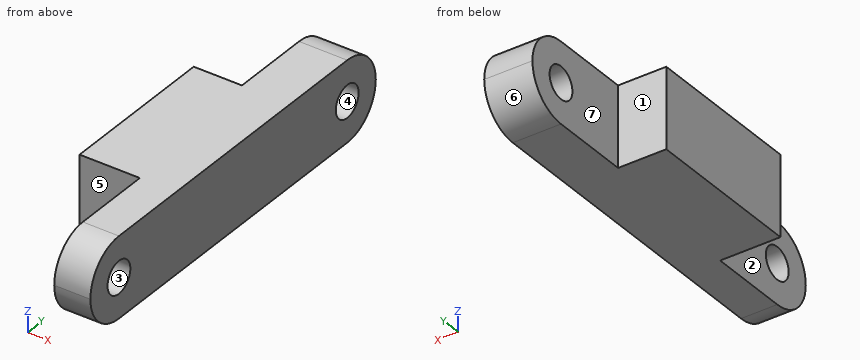
from build123d import *

# Parameters (mm, degrees)
SKETCH1_W           = 12
SKETCH1_H           = 50
BOSS_EXTRUDE1_DEPTH = 10
SKETCH2_W           = 7.5
SKETCH2_H           = 15
SKETCH2_W_2         = 6
CUT_EXTRUDE1_DEPTH  = 10
SKETCH3_R           = 2
CUT_EXTRUDE2_DEPTH  = 10
FILLET1_R           = 5


with BuildPart() as part:
    # Sketch1 → Boss-Extrude1 (new body)
    with BuildSketch(Plane.XY):
        Rectangle(SKETCH1_W, SKETCH1_H)
    extrude(amount=BOSS_EXTRUDE1_DEPTH)

    # Sketch2 → Cut-Extrude1 (cut)
    with BuildSketch(Plane.XY.offset(10)):
        with Locations((-2.25, -17.5)):
            Rectangle(SKETCH2_W, SKETCH2_H)
        with Locations((-3, 17.5)):
            Rectangle(SKETCH2_W_2, SKETCH2_H)
    extrude(amount=-CUT_EXTRUDE1_DEPTH, mode=Mode.SUBTRACT)

    # Sketch3 → Cut-Extrude2 (cut)
    with BuildSketch(Plane.ZY):
        with Locations(Location((5, 20, 0), (0, 0, 270))):
            Circle(SKETCH3_R)
        with Locations(Location((5, -20, 0), (0, 0, 270))):
            Circle(SKETCH3_R)
    extrude(amount=-CUT_EXTRUDE2_DEPTH, mode=Mode.SUBTRACT)

    # Fillet1
    fillet1_edges = [part.edges().sort_by_distance(p)[0] for p in [
        (3.75, -25, 0),
        (3.75, -25, 10),
        (3, 25, 0),
        (3, 25, 10),
    ]]
    fillet(fillet1_edges, radius=FILLET1_R - 0.0001)  # a hair under: the kernel refuses the full size


solid = part.part
Work out the finished part from the listing and answer in its coordinate system (mm). Face numbers are marked on the shaded views. A direction names the side the tool comes from. Coordinates: 2 decimals unless noted, no trailing zeros. Loops run counter-clockwise (first coordinate to the right, second up) from the corner with the lowest first, then second, coordinate; pieces in that order, holes last. Notation, with made-up numbers: M 48,23.5 L 65,23.5 A21 cw 65,27.5 Z; hole C 66,-26 d4. An arc over 180 degrees is marked long. Answer in a Markdown table with one row per item. Add a question column.
1. A tool of negligible diameter and unlimited length cuts with its end or side. For the marked faces 5, 6 and 7, from which of +Z, -Z, +X, -X, +Y, -Y can it reach the whole face along a straight path? Write none if from no direction.
2. Find section A-A, the plane x = 3. State how many separate pieces and enclosed holes the cut face has, then the cut area to 3 significant figures.
3. Find section C-C, the plane y = -19. Write down the section's boundary in (x, z).
4. Consider L1, parallel to Z at x = 1.75, y = 20; L2, parallel to Y at x = 2, z = 4; L3, parallel to Y at x = -2.5, z = 5.75. Determine where each line is inside the solid, lowest interval first.
5. Flat-ended cylindrical pins translate along their axes: P1, Ø4, axis at x = -2, z = 3, coming from the -Y side; P2, Ø3.5, axis at y = -20, z = 5, coming from the +X side; P3, Ø3, axis at x = -4, z = 7, coming from the +Y side. Find the tip coordinate at first contact, or state that the pin passes through.
6. Find section D-D, the plane x = -5.5. Write down the section's boundary in (y, z).
7. The mould has two halves that part along Y. Classify the marked faces 1, 2, 3 and 4: pulls with the +Y half, pulls with the -Y half, needs draft (parallel to the pull), parting line crosses it, or undercut.
8. Find section B-B, the plane z = 3.75. Write down the section's boundary in (x, y), then the cut area to 3 significant figures.
Reported:
| question | item | result |
|---|---|---|
| 1 | face 5 | +Z, -Z, -X, -Y |
| 1 | face 6 | -Z, +X, -X, +Y |
| 1 | face 7 | +Z, -Z, -X, +Y |
| 2 | separate pieces | 1 |
| 2 | enclosed holes | 2 |
| 2 | area | 453 mm^2 |
| 3 | outline | M 1.5,0 L 6,0 L 6,3.27 L 1.5,3.27 Z; M 1.5,6.73 L 6,6.73 L 6,10 L 1.5,10 Z |
| 4 | L1 | z = 0 to 3, 7 to 10 |
| 4 | L2 | y = -24.9 to -21.73, -18.27 to 18.27, 21.73 to 24.9 |
| 4 | L3 | y = -10 to 10 |
| 5 | P1 | stops at y = -10 |
| 5 | P2 | passes through |
| 5 | P3 | stops at y = 10 |
| 6 | outline | M -10,0 L 10,0 L 10,10 L -10,10 Z |
| 7 | face 1 | pulls with the +Y half |
| 7 | face 2 | needs draft |
| 7 | face 3 | undercut |
| 7 | face 4 | undercut |
| 8 | outline | M -6,-10 L 1.5,-10 L 1.5,-18.44 L 6,-18.44 L 6,18.44 L 0,18.44 L 0,10 L -6,10 Z; M 0,21.56 L 6,21.56 L 6,24.84 L 0,24.84 Z; M 1.5,-24.84 L 6,-24.84 L 6,-21.56 L 1.5,-21.56 Z |
| 8 | area | 363 mm^2 |
